Geometry: final body of the model. Coordinates: model frame, mm. Coordinates: 2 decimals unless noted, no trailing zeros. Loops run counter-clockwise (first coordinate to the right, second up) from the corner with the lowest first, then second, coordinate; pieces in that order, holes last. Notation, with made-up numbers: M 76,46 L 99,46 A24 ccw 99,76 Z; hole C 34.25,-14.5 d11. An arc over 180 degrees is marked long. Write item = value, one per line. Start each with the question number.
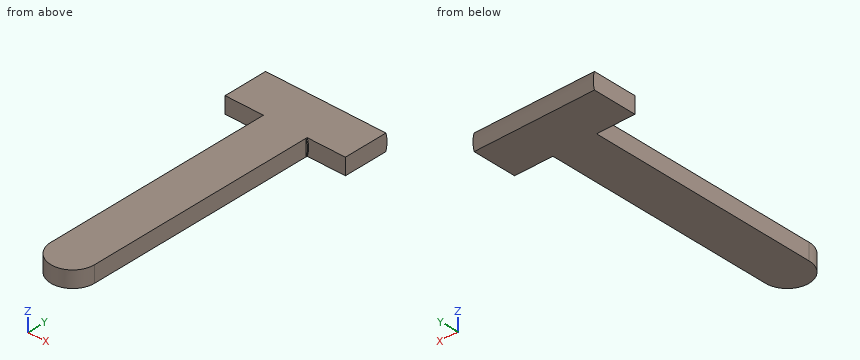
```python
from build123d import *

# Parameters (mm, degrees)
EXTRUSION1_DEPTH = 1.5
EXTRUSION2_DEPTH = 0.1
EXTRUSION3_DEPTH = 11


with BuildPart() as part:
    # Esquisse1 → Extrusion1 (new body)
    with BuildSketch(Plane.XY):
        with BuildLine():
            Line((-5.5, 0), (5.5, 0))
            Line((5.5, 0), (5.5, -4))
            Line((5.5, -4), (2, -4))
            Line((2, -4), (2, -25))
            ThreePointArc((2, -25), (0, -27), (-2, -25))
            Line((-2, -25), (-2, -4))
            Line((-2, -4), (-5.5, -4))
            Line((-5.5, -4), (-5.5, 0))
        make_face()
    extrude(amount=EXTRUSION1_DEPTH)

    # Esquisse2 → Extrusion2 (add)
    with BuildSketch(Plane.XZ.offset(4)):
        with BuildLine():
            Line((-2, 1.5), (-2, 0))
            ThreePointArc((-2, 0), (-2.136000936, 0.75), (-2, 1.5))
        make_face()
        with BuildLine():
            Line((2, 1.5), (2, 0))
            ThreePointArc((2, 0), (2.136000936, 0.75), (2, 1.5))
        make_face()
    extrude(amount=EXTRUSION2_DEPTH)

    # Esquisse3 → Extrusion3 (add)
    with BuildSketch(Plane.ZY.offset(5.5)):
        with BuildLine():
            Line((1.5, 0), (0, 0))
            ThreePointArc((0, 0), (0.75, 0.115151996), (1.5, 0))
        make_face()
    extrude(amount=-EXTRUSION3_DEPTH)


solid = part.part
```
Item 1: Line query: line 1 (X direction, y = -4.5, z = 0.85); line 2 (Y direction, x = 0, z = 0.65); line 3 (Y direction, x = 3.25, z = 0.7). Output: solid intervals per line, ascending. Write a range as from..to.
Item 2: First-contact query: pin 1 (0.8 mm diameter, centred on y = -12, z = 1, fed in from +X); pin 2 (0.8 mm diameter, centred on y = -10.5, z = 1, fed in from -X); pin 3 (0.5 mm diameter, centred on x = -4, z = 1, fed in from -Y). Flat tips, straight axial feed; report the tip coordinate or a pass-through.
Item 3: Section query C-C (x = 4.75). Return the cut outline in (y, z), plus the area to 3 significant figures.
Item 4: Section query B-B (y = -14). Return the cut outline in (x, z), plus the area to 3 significant figures.
Item 5: Section query A-A (z = 0.6). Return the cut outline in (x, y), plus the area to 3 significant figures.
Verdict:
q1.line_1 = -2..2
q1.line_2 = -27..0.11
q1.line_3 = -4..0.11
q2.pin_1 = 2
q2.pin_2 = -2
q2.pin_3 = -4
q3.outline = M -4,0 L 0,0 A2.5 ccw 0,1.5 L -4,1.5 Z
q3.area = 6.12 mm2
q4.outline = M -2,0 L 2,0 L 2,1.5 L -2,1.5 Z
q4.area = 6.00 mm2
q5.outline = M -5.5,-4 L -2.13,-4 L -2.13,-4.1 L -2,-4.1 L -2,-25 A2 ccw 2,-25 L 2,-4.1 L 2.13,-4.1 L 2.13,-4 L 5.5,-4 L 5.5,0.11 L -5.5,0.11 Z
q5.area = 136 mm2
